from build123d import *

# Parameters (mm, degrees)
MODEL_R         = 1.5
MODEL_R_2       = 11
MODEL_R_3       = 3
EXTRUDE_1_DEPTH = 3


with BuildPart() as part:
    # Model → 凸台-拉伸1 (new body)
    with BuildSketch(Plane.XY):
        with BuildLine():
            ThreePointArc((39.503035275, -6.285714286), (49.655052701, 11.819164878), (69.130311731, 19))
            Line((69.130311731, 19), (250.869688269, 19))
            ThreePointArc((250.869688269, 19), (270.344947299, 11.819164878), (280.496964725, -6.285714286))
            ThreePointArc((280.496964725, -6.285714286), (324.480836134, -39.748234018), (359.911012126, 2.666666667))
            ThreePointArc((359.911012126, 2.666666667), (365.260583322, 17.662601021), (379.866518188, 24))
            Line((379.866518188, 24), (380, 24))
            ThreePointArc((380, 24), (383.535533906, 25.464466094), (385, 29))
            Line((385, 29), (385, 38.996919308))
            ThreePointArc((385, 38.996919308), (376.213203436, 60.210122744), (355, 68.996919308))
            Line((355, 68.996919308), (0.221994544, 68.996919308))
            ThreePointArc((0.221994544, 68.996919308), (-28.062276703, 57.281190556), (-39.778005456, 28.996919308))
            Line((-39.778005456, 28.996919308), (-39.995311376, 0.612427911))
            Line((-39.995311376, 0.612427911), (-40, 0))
            ThreePointArc((-40, 0), (-3.152664667, -39.875565269), (39.503035275, -6.285714286))
        make_face()
        with Locations((-6, -24.5)):
            Circle(MODEL_R, mode=Mode.SUBTRACT)
        with Locations((6, -24.5)):
            Circle(MODEL_R, mode=Mode.SUBTRACT)
        with Locations((0, -14)):
            Circle(MODEL_R, mode=Mode.SUBTRACT)
        with Locations((-14, 0)):
            Circle(MODEL_R, mode=Mode.SUBTRACT)
        Circle(MODEL_R_2, mode=Mode.SUBTRACT)
        with Locations((14, 0)):
            Circle(MODEL_R, mode=Mode.SUBTRACT)
        with Locations((0, 14)):
            Circle(MODEL_R, mode=Mode.SUBTRACT)
        with Locations((314, -24.5)):
            Circle(MODEL_R, mode=Mode.SUBTRACT)
        with Locations((326, -24.5)):
            Circle(MODEL_R, mode=Mode.SUBTRACT)
        with Locations((320, -14)):
            Circle(MODEL_R, mode=Mode.SUBTRACT)
        with Locations((306, 0)):
            Circle(MODEL_R, mode=Mode.SUBTRACT)
        with Locations((320, 0)):
            Circle(MODEL_R_2, mode=Mode.SUBTRACT)
        with Locations((334, 0)):
            Circle(MODEL_R, mode=Mode.SUBTRACT)
        with Locations((320, 14)):
            Circle(MODEL_R, mode=Mode.SUBTRACT)
        with Locations((-14, 41.5)):
            Circle(MODEL_R, mode=Mode.SUBTRACT)
        with Locations((-2, 41.5)):
            Circle(MODEL_R, mode=Mode.SUBTRACT)
        with Locations((104, 41.5)):
            Circle(MODEL_R, mode=Mode.SUBTRACT)
        with Locations((116, 41.5)):
            Circle(MODEL_R, mode=Mode.SUBTRACT)
        with Locations((54.983182049, 63.996919308)):
            Circle(MODEL_R_3, mode=Mode.SUBTRACT)
        with Locations((122, 58.496919308)):
            Circle(MODEL_R, mode=Mode.SUBTRACT)
        with Locations((134, 58.496919308)):
            Circle(MODEL_R, mode=Mode.SUBTRACT)
        with Locations((196, 36.5)):
            Circle(MODEL_R_3, mode=Mode.SUBTRACT)
        with Locations((224, 41.5)):
            Circle(MODEL_R, mode=Mode.SUBTRACT)
        with Locations((236, 41.5)):
            Circle(MODEL_R, mode=Mode.SUBTRACT)
        with Locations((344, 18.5)):
            Circle(MODEL_R, mode=Mode.SUBTRACT)
        with Locations((356, 18.5)):
            Circle(MODEL_R, mode=Mode.SUBTRACT)
        with Locations((186, 58.496919308)):
            Circle(MODEL_R, mode=Mode.SUBTRACT)
        with Locations((198, 58.496919308)):
            Circle(MODEL_R, mode=Mode.SUBTRACT)
        with Locations((215, 63.996919308)):
            Circle(MODEL_R_3, mode=Mode.SUBTRACT)
        with Locations((255, 63.996919308)):
            Circle(MODEL_R_3, mode=Mode.SUBTRACT)
    extrude(amount=EXTRUDE_1_DEPTH)


solid = part.part
Design review of the part built by this model. Coordinates are the model's own, in mm. A direction names the side the tool comes from. Give positions to 0.01 mm unless a question says otherwise; leave off trailing zeros. Loops run counter-clockwise (first coordinate to the right, second up) from the corner with the lowest first, then second, coordinate; pieces in that order, holes last. Notation, with made-up numbers: (15.5, 40.5) - (22.5, 40.5) arc R19 ccw to (22.5, 67.5) - close; hole circle Ø7 at (-31, 3.25). An arc over 180 degrees is marked (long way). Use CSV: the item, a comma, the result in double quotes. Start each with the question number.
1. Add section B-B (z = 0.85). Count the separate pieces of the cut face and the enclosed holes in it, plus the area to 3 significant figures.
2. Draft analysis for pull direction Y (two halves, no side actions). For faces 1 (the cylindrical face through (-2.38, -10.74, 1.48)), 2 (the cylindrical face through (309, 0, 1)), 3 (the flat face through (170, 27, 3)), 4 (the cylindrical face through (270.12, 12.01, 1.48)), state which applies: released by +Y, released by -Y, zero draft, split by the parting line, or undercut.
3. Add section A-A (y = -33). State the section outline as (x, z) points.
4. Wall thickness on L1, parallel to Y at x = 186, z = 1.6; L2, parallel to Y at x = 315, z = 1.5; L3, parallel to Y at x = 224, z = 0.7: over which ranges is each line inside the solid? List them lowest first.
5. Insertion check: P1, Ø0.9, axis at x = 144.5, z = 1, coming from the -Y side; P2, Ø1.5, axis at y = 35, z = 0.5, coming from the -X side. Each pin has a flat end and moves straight along its axis. Give the tip position at first contact, or say it passes through.
6. Machinability: for faces 5 (the cylindrical face through (49.4, 11.6, 1.5)), 6 (the flat face through (170, 27, 0)), which of the approach directions +Z, -Z, +X, -X, +Y, -Y give a long, thin tool a straight path to every point of the face, cutting with its end or side? Answer none if there is none.
Results found:
1,separate pieces,"1"
1,enclosed holes,"30"
1,area,"28,000 mm²"
2,face 1,"undercut"
2,face 2,"undercut"
2,face 3,"zero draft"
2,face 4,"released by -Y"
3,outline,"(-22.61, 0) - (22.61, 0) - (22.61, 3) - (-22.61, 3) - close; (297.39, 0) - (342.61, 0) - (342.61, 3) - (297.39, 3) - close"
4,L1,"y = 19 to 57, 60 to 69"
4,L2,"y = -39.69 to -25.62, -23.38 to -9.8, 9.8 to 69"
4,L3,"y = 19 to 40, 43 to 69"
5,P1,"stops at y = 19"
5,P2,"stops at x = -39.43"
6,face 5,"+Z, -Z, -Y"
6,face 6,"-Z, +X, -X, +Y, -Y"
